Autodesk Inventor part; units mm, degrees
ref_plane "YZ Plane" through (0, 0, 0) normal (1, 0, 0) x (0, 1, 0)
ref_plane "XY Plane" through (0, 0, 0) normal (0, 0, 1) x (1, 0, 0)
sketch "Sketch1" plane through (0, 0, 0) normal (0, 0, 1) x (1, 0, 0)
  line L0 (0, -11) -> (-10.5, -11)
  line L1 (-10.5, -11) -> (-10.5, 31)
  line L2 (-10.5, 31) -> (10.5, 31)
  line L3 (10.5, 31) -> (10.5, -11)
  line L4 (10.5, -11) -> (0, -11)
  line L5 (10.5, 10) -> (0, 10)
  line L6 (0, 0) -> (0, 10)
  circle A0 centre (0, 0) radius 42.5
  dimension "d1" = 42
  dimension "d28" = 21
  dimension "d76" = 10
  dimension "d77" = 10.5
  dimension "d78" = 85
extrude "Extrusion6" add sketch "Sketch1" along normal blind 5
sketch "Sketch9" plane through (0, 0, 5) normal (0, 0, 1) x (1, 0, 0)
  line L0 (10.5, -11) -> (-10.5, -11)
  line L1 (0, -11) -> (0, -14)
  line L2 (0, -14) -> (-5, -14)
  circle A0 centre (-5, -14) radius 3
  line L3 (0, -14) -> (5, -14)
  circle A1 centre (5, -14) radius 3
  line L4 (-10.5, -11) -> (-10.5, 31)
  line L5 (-10.5, 10) -> (10.5, 10)
  line L6 (10.5, 31) -> (-10.5, 31)
  line L7 (0, 31) -> (0, 34)
  line L8 (0, 34) -> (-5, 34)
  circle A2 centre (-5, 34) radius 3
  line L9 (0, 34) -> (5, 34)
  circle A3 centre (5, 34) radius 3
  dimension "d79" = 3
  dimension "d80" = 5
  dimension "d81" = 6
  dimension "d82" = 5
  dimension "d83" = 6
extrude "Extrusion12" cut sketch "Sketch9" against normal through all contours A2 | A1 | A0 | A3
sketch "Sketch10" plane through (0, 0, 5) normal (0, 0, 1) x (1, 0, 0)
  line L0 (-10.5, 31) -> (-10.5, 38.5)
  circle A0 centre (0, 0) radius 39.9061
  line L1 (-10.5, -11) -> (-10.5, -18.5)
  arc A1 (-21.272, 0) -> (21.272, 0) centre (0, 0) ccw
  arc A2 (-21.272, 0) -> (-10.5, 31) centre (-71.284, 34.75) ccw
  line L2 (10.5, 31) -> (10.5, 38.5)
  arc A3 (10.5, 31) -> (21.272, 0) centre (71.284, 34.75) ccw
  dimension "d86" = 7.5
  dimension "d87" = 79.8123
  dimension "d88" = 7.5
extrude "Extrusion13" add sketch "Sketch10" along normal blind 35 contours A2 A1 A3 L2 A0 L0 picked at (-28.5299, 15.6602)
sketch "Sketch11" plane through (0, 0, 40) normal (0, 0, 1) x (1, 0, 0)
  line L0 (0, 0) -> (0, -30)
  circle A0 centre (0, -30) radius 1.75
  circle A1 centre (21.2132, -21.2132) radius 1.75
  circle A2 centre (30, 0) radius 1.75
  circle A3 centre (21.2132, 21.2132) radius 1.75
  circle A4 centre (0, 30) radius 1.75
  circle A5 centre (-21.2132, 21.2132) radius 1.75
  circle A6 centre (-30, 0) radius 1.75
  circle A7 centre (-21.2132, -21.2132) radius 1.75
  dimension "d91" = 30
  dimension "d92" = 3.5
  dimension "d95" = 360
extrude "Extrusion14" cut sketch "Sketch11" against normal through all contours A0 | A1 | A2 | A3 | A5 | A6 | A7
sketch "Sketch12" plane through (0, 0, 40) normal (0, 0, 1) x (1, 0, 0)
  line L0 (0, 0) -> (0, -39.9061)
  arc A0 (-10.5, 38.5) -> (10.5, 38.5) centre (0, 0) ccw
ref_plane "Work Plane2" through (0, -39.9061, 40) normal (0, 1, 0) x (-1, 0, 0)
sketch "Sketch13" plane through (0, -39.9061, 40) normal (0, 1, 0) x (-1, 0, 0)
  line L0 (-0.0018, 0) -> (-0.0018, -10)
  line L1 (-0.0018, -10) -> (-4.0018, -10)
  line L2 (-4.0018, -10) -> (-4.0018, -14)
  line L3 (-4.0018, -14) -> (3.9982, -14)
  line L4 (3.9982, -14) -> (3.9982, -10)
  line L5 (3.9982, -10) -> (-0.0018, -10)
  point P0 (0, -40)
  dimension "d99" = 10
  dimension "d100" = 4
  dimension "d101" = 4
  dimension "d102" = 8
extrude "Extrusion15" cut sketch "Sketch13" along normal blind 15
pattern_circular "Circular Pattern2" count 8 over 360 about axis through (0, 0, 5) along (0, 0, 1) of "Extrusion15"
ref_plane "Work Plane3" through (10.5, 38.5, 40) normal (0, -1, 0) x (-1, 0, 0)
sketch "Sketch14" plane through (10.5, 38.5, 40) normal (0, -1, 0) x (-1, 0, 0)
  line L0 (0, 35) -> (5.5, 35)
  line L1 (-10.772, 35) -> (-10.772, 0)
  line L2 (-10, 35) -> (-8, 35) construction
  line L3 (-10, 33) -> (0, 33)
  line L4 (-10, 33) -> (-10, 13)
  line L5 (-9.941, 10) -> (-9.941, 14)
  line L6 (-10, 33) -> (10, 33) construction
  line L7 (-10, 13) -> (0, 13)
  line L8 (0, 13) -> (0, 33)
  line L9 (0, 35) -> (0, 0)
  line L10 (21, 35) -> (21, 0)
  line L11 (21, 33) -> (31, 33)
  line L12 (31, 33) -> (31, 13)
  line L13 (31, 13) -> (21, 13)
  line L14 (21, 13) -> (21, 33)
  point P0 (10.5, 40)
  dimension "d109" = 2
  dimension "d111" = 20
  dimension "d112" = 90
  dimension "d113" = 10
  dimension "d114" = 20
extrude "Extrusion16" cut sketch "Sketch14" along normal blind 7.5
sketch "Sketch15" plane through (10.5, 31, 40) normal (0, 1, 0) x (1, 0, 0)
  line L0 (-21, 13) -> (-21, 0)
  line L1 (-31, 13) -> (-31, 33)
  line L2 (-21, 33) -> (-21, 13)
  line L3 (0, 35) -> (0, 33)
  line L4 (10, 13) -> (0, 13)
  line L5 (0, 33) -> (10, 33)
  circle A0 centre (5, 23) radius 1.5
  circle A1 centre (-26, 23) radius 1.5
  point P0 (-10.5, 40)
  dimension "d118" = 3
  dimension "d119" = 3
extrude "Extrusion17" cut sketch "Sketch15" against normal blind 5
properties part number "rotacion2_top"
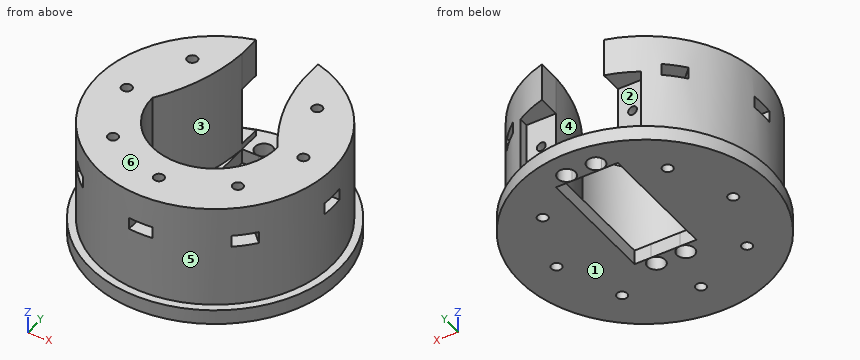
Check sheet for the modelled part. Datum: model origin and axes. Units: mm. Face numbers are marked on the shaded views. A direction names the side the tool comes from. Round coordinates to 2 decimals unless told otherwise and drop trailing zeros. Order: outer loops, then holes, each group sorted by start corner. A loop starts at its lowest first (then second) coordinate and runs counter-clockwise, first axis right, second up. Notation, with made-up numbers: (0.25, -13.5) -> (28.25, -13.5) arc R19 cw to (28.25, -3.5) -> close; hole circle Ø5 at (2, -10.75). An arc over 180 degrees is marked (long way). One line per item, written item: value. Start each with the question number.
Q1. Gauge pin test, flat ends, axial feed: pin 1 Ø4.5 at (y, z) = (-33, 28) entering from +X; pin 2 Ø2.5 at (y, z) = (1.5, 2.5) entering from +X; pin 3 Ø3 at (x, y) = (-30, 0) entering from -Z; pin 4 Ø12 at (x, z) = (-15, 27.5) entering from +Y. Record the tip position at first contact, or that the pin passes through.
Q2. Cross-section at A-A (y = -6). Record the boundary of the cut face in (x, z).
Q3. Cross-section at C-C (z = 36.5). Record the boundary of the cut face in (x, y), and give its area (3 significant figures).
Q4. Mould release check, pull along X, two halves, no side actions. Record for the marked faces 4, 5 and 6: pulls with the +X half, pulls with the -X half, needs draft (parallel to the pull), parting line crosses it, or undercut.
Q5. Cross-section at D-D (y = -37). Record the boundary of the cut face in (x, z).
Q6. Set-up check for the marked faces 1, 2 and 3: record each of +Z, -Z, +X, -X, +Y, -Y from which the full face is reachable in a straight line by a thin tool's end or side.
Q7. Cross-section at B-B (x = 27). Record the boundary of the cut face in (y, z), and give its area (3 significant figures).
Q8. Thickness scan on line 1 (X direction, y = 20.5, z = 20.5); line 2 (X direction, y = -14, z = 2.3); line 3 (Z direction, x = 19, y = -8.5). Record the ranges inside material, lowest first.
Completed:
1. pin 1: stops at x = 25.25
1. pin 2: stops at x = 42.5
1. pin 3: passes through
1. pin 4: stops at y = 38.5
2. outline: (-42.07, 0) -> (-10.5, 0) -> (-10.5, 5) -> (-20.41, 5) -> (-20.41, 40) -> (-39.45, 40) -> (-39.45, 5) -> (-42.07, 5) -> close; (10.5, 0) -> (42.07, 0) -> (42.07, 5) -> (39.45, 5) -> (39.45, 40) -> (20.41, 40) -> (20.41, 5) -> (10.5, 5) -> close
3. outline: (-21.27, 0) arc R60.9 ccw to (-10.5, 31) -> (-10.5, 38.5) arc R39.91 ccw (long way) to (10.5, 38.5) -> (10.5, 31) arc R60.9 ccw to (21.27, 0) arc R21.27 cw to start; hole circle Ø3.5 at (-30, 0); hole circle Ø3.5 at (-21.21, -21.21); hole circle Ø3.5 at (-21.21, 21.21); hole circle Ø3.5 at (0, -30); hole circle Ø3.5 at (21.21, -21.21); hole circle Ø3.5 at (21.21, 21.21); hole circle Ø3.5 at (30, 0)
3. area: 3,160 mm²
4. face 4: undercut
4. face 5: parting line crosses it
4. face 6: needs draft
5. outline: (-20.91, 0) -> (20.91, 0) -> (20.91, 5) -> (14.95, 5) -> (14.95, 40) -> (-14.95, 40) -> (-14.95, 5) -> (-20.91, 5) -> close; hole (-4, 26) -> (4, 26) -> (4, 30) -> (-4, 30) -> close
6. face 1: -Z, +X, -X, +Y, -Y
6. face 2: +Y
6. face 3: +Z
7. outline: (-32.82, 0) -> (32.82, 0) -> (32.82, 5) -> (29.39, 5) -> (29.39, 26) -> (21.35, 26) -> (21.35, 30) -> (29.39, 30) -> (29.39, 40) -> (-29.39, 40) -> (-29.39, 30) -> (-21.34, 30) -> (-21.34, 26) -> (-29.39, 26) -> (-29.39, 5) -> (-32.82, 5) -> close; hole (-4, 26) -> (4, 26) -> (4, 30) -> (-4, 30) -> close
7. area: 2,290 mm²
8. line 1: x = -34.24 to -22.81, -19.62 to -12.08, 12.08 to 19.62, 22.81 to 34.24
8. line 2: x = -40.13 to -8, -2 to 2, 8 to 40.13
8. line 3: z = 0 to 5
